Source: CAD feature listing. Evaluate the final solid. Frame: model axes, mm. Face numbers are marked on the shaded views. A direction names the side the tool comes from. Coordinates: 2 decimals unless noted, no trailing zeros. Write each loop counter-clockwise with the first axis right and the second up, starting at its lowest first coordinate (ties: lowest second). Pieces come first, ordered by that corner, then holes. Notation, with made-up numbers: M 25,43 L 54,43 A17 ccw 54,68 Z; hole C -31.5,-40 d2. An arc over 180 degrees is marked long. Write item = value, one per line. Start each with the question number.
1. Section query A-A (y = 0). Give the number of separate pieces and of enclosed holes in the cut face, then the cut area to 3 significant figures.
2. Section query C-C (z = 20). Output: boundary loops of the cut face in (x, y), then the cut area to 3 significant figures.
3. Pull-direction query (Y, two-part tool) for the marked faces 4, 5 and 6; classes: pulls with the +Y half, pulls with the -Y half, needs draft (parallel to the pull), parting line crosses it, or undercut.
4. Access query for the marked faces 1, 2 and 3. Directions: +Z, -Z, +X, -X, +Y, -Y. A direction counts if a zero-diameter tool reaches every point of the face in a straight line with its end or side. Return the directions, or none.
5. Section query B-B (z = 6.5). Output: boundary loops of the cut face in (x, y).
6. Pin query (flat end, axial travel): pin 1 Ø5 at (x, y) = (-3, -0.5) entering from -Z; pin 2 Ø2 at (x, z) = (-5, 23) entering from +Y; pin 3 Ø6 at (y, z) = (11, 4) entering from +X. Return the tip coordinate at first contact, or that it passes through.
7. Line query: line 1 along X through (y, z) = (-3, 9.25); line 2 along Z through (x, y) = (19, 10); line 3 along Z through (x, y) = (-3.5, -3). Output: solid intervals per line, ascending.
```python
from build123d import *

# Parameters (mm, degrees)
SKETCH1_R           = 22.5
SKETCH1_R_2         = 2
BOSS_EXTRUDE1_DEPTH = 8
SKETCH2_R           = 11
SKETCH2_R_2         = 4
BOSS_EXTRUDE2_DEPTH = 20
FILLET1_R           = 10
CUT_EXTRUDE1_START  = -8
CUT_EXTRUDE1_DEPTH  = 35.385138905


with BuildPart() as part:
    # Sketch1 → Boss-Extrude1 (new body)
    with BuildSketch(Plane.XY):
        Circle(SKETCH1_R)
        with Locations((-13.75, 0)):
            Circle(SKETCH1_R_2, mode=Mode.SUBTRACT)
        with Locations((13.75, 0)):
            Circle(SKETCH1_R_2, mode=Mode.SUBTRACT)
        Polygon((0, 9.814954576), (-8.5, 4.907477288), (-8.5, -4.907477288), (0, -9.814954576), (8.5, -4.907477288), (8.5, 4.907477288), align=None, mode=Mode.SUBTRACT)
    extrude(amount=BOSS_EXTRUDE1_DEPTH)

    # Sketch2 → Boss-Extrude2 (add)
    with BuildSketch(Plane.XY.offset(8)):
        Circle(SKETCH2_R)
        Circle(SKETCH2_R_2, mode=Mode.SUBTRACT)
    extrude(amount=BOSS_EXTRUDE2_DEPTH)

    # Fillet1
    # the kernel refuses this fillet: 10 mm, written as the material it adds along each edge
    with BuildSketch(Plane(origin=(0, 0, 8), x_dir=(1, 0, 0), z_dir=(0, -1, 0))) as fillet1_piece_1_section:
        with BuildLine():
            CenterArc((11 + FILLET1_R, FILLET1_R), FILLET1_R, 180, 90)
            Line((11, FILLET1_R), (11, 0))
            Line((11, 0), (11 + FILLET1_R, 0))
        make_face()
    fillet1_piece_1 = revolve(axis=Axis((0, 0, 8), (0, 0, 1)), mode=Mode.PRIVATE)
    fillet1_piece_1 = fillet1_piece_1 - Plane(origin=(-13.75, 0, 8.218261163), x_dir=(1, 0, 0), z_dir=(0, 0, -1)) * Cylinder(2, 84, mode=Mode.PRIVATE)
    fillet1_piece_1 = fillet1_piece_1 - Plane(origin=(13.75, 0, 8.218261163), x_dir=(1, 0, 0), z_dir=(0, 0, -1)) * Cylinder(2, 84, mode=Mode.PRIVATE)
    add(fillet1_piece_1)

    # Sketch3 → Cut-Extrude1 (cut, through all)
    with BuildSketch(Plane(origin=(0, 0, 0), x_dir=(-1, 0, 0), z_dir=(0, 0, -1)).offset(CUT_EXTRUDE1_START)):
        Polygon((-13.75, 4.041451884), (-17.25, 2.020725942), (-17.25, -2.020725942), (-13.75, -4.041451884), (-10.25, -2.020725942), (-10.25, 2.020725942), align=None)
        Polygon((13.75, 4.041451884), (10.25, 2.020725942), (10.25, -2.020725942), (13.75, -4.041451884), (17.25, -2.020725942), (17.25, 2.020725942), align=None)
    extrude(amount=-CUT_EXTRUDE1_DEPTH, mode=Mode.SUBTRACT)


solid = part.part
```
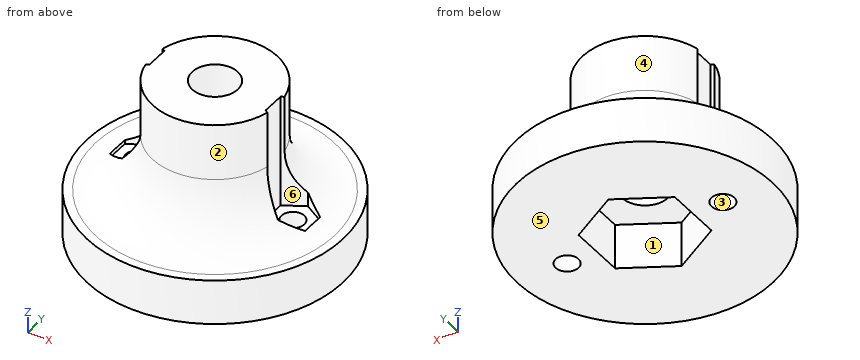
Results are:
q1.separate_pieces = 4
q1.enclosed_holes = 0
q1.area = 412 mm^2
q2.outline = M -10.75,-2.31 A11 ccw 10.75,-2.31 L 10.25,-2.02 L 10.25,2.02 L 10.75,2.31 A11 ccw -10.75,2.31 L -10.25,2.02 L -10.25,-2.02 Z; hole C 0,0 d8
q2.area = 324 mm^2
q3.face_4 = pulls with the +Y half
q3.face_5 = needs draft
q3.face_6 = undercut
q4.face_1 = -Z
q4.face_2 = +Z, -Y
q4.face_3 = +Z, -Z
q5.outline = C 0,0 d45; hole C -13.75,0 d4; hole M -8.5,-4.91 L 0,-9.81 L 8.5,-4.91 L 8.5,4.91 L 0,9.81 L -8.5,4.91 Z; hole C 13.75,0 d4
q6.pin_1 = 8
q6.pin_2 = 10.25
q6.pin_3 = 21.03
q7.line_1 = -15.88 to -15.55, -11.95 to -2.65, 2.65 to 11.95, 15.55 to 15.88
q7.line_2 = 0 to 8
q7.line_3 = 8 to 28
